from build123d import *

# Parameters (mm, degrees)
SKETCH1_W           = 30
SKETCH1_H           = 75
BOSS_EXTRUDE1_DEPTH = 12
CUT_EXTRUDE1_DEPTH  = 12
LPATTERN1_COUNT     = 3
LPATTERN1_PITCH     = 20
BOUNDARY2_START     = -15
BOUNDARY2_DEPTH     = 5


# Read off the part's stored shape, not the designer's step: Boundary2
with BuildPart() as part:
    # Sketch1 → Boss-Extrude1 (new body)
    with BuildSketch(Plane(origin=(0, 0, 0), x_dir=(1, 0, 0), z_dir=(0, 1, 0))):
        with Locations((15, 37.5)):
            Rectangle(SKETCH1_W, SKETCH1_H)
    extrude(amount=BOSS_EXTRUDE1_DEPTH)

    # Sketch3 → Cut-Extrude1 (cut)
    with BuildSketch(Plane(origin=(0, 0, 0), x_dir=(1, 0, 0), z_dir=(0, 1, 0))):
        Polygon((0, 5), (22.5, 12.5), (0, 20), align=None)
    cut_extrude1 = extrude(amount=CUT_EXTRUDE1_DEPTH, mode=Mode.SUBTRACT)

    # LPattern1: Cut-Extrude1 ×3
    with Locations(*[(0, 0, -i * LPATTERN1_PITCH) for i in range(1, LPATTERN1_COUNT)]):
        add(cut_extrude1, mode=Mode.SUBTRACT)

    # Boundary2 outline → Boundary2 (add)
    with BuildSketch(Plane.XY.offset(BOUNDARY2_START)):
        Polygon((30, 0), (25, 0), (30, -2), align=None)
    extrude(amount=BOUNDARY2_DEPTH)


solid = part.part
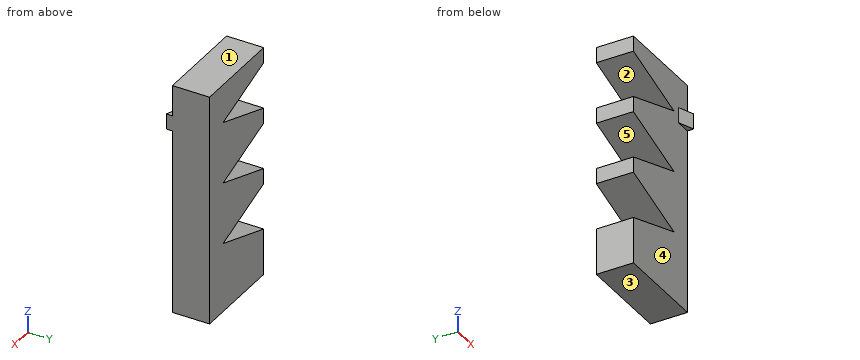
Input: part model. Units: mm. Frame: model coordinates. Face numbers are marked on the shaded views. A direction names the side the tool comes from. Coordinates: 2 decimals unless noted, no trailing zeros. Loops run counter-clockwise (first coordinate to the right, second up) from the corner with the lowest first, then second, coordinate; pieces in that order, holes last. Notation, with made-up numbers: (-5.75, 39) - (15.25, 39) arc R18 ccw to (15.25, 61) - close; hole circle Ø2 at (-8, -10.75). An arc over 180 degrees is marked (long way). Answer in a Markdown table with one row per item. Add a question column.
Item 1: Section query D-D on z = -11. Return the cut outline in (x, y), then the cut area to 3 significant figures.
Item 2: Mould query, pull axis Z, two halves, no side actions, for the marked faces 3, 4 and 5. Classes: released by +Z, released by -Z, zero draft, split by the parting line, or undercut.
Item 3: Contact query for flat-ended pins moving along their axis: P1, Ø4, axis at x = 26, y = 3.5, coming from the +Z side; P2, Ø1, axis at x = 27, y = -1, coming from the +Z side; P3, Ø4, axis at x = 4, z = -22, coming from the -Y side; P4, Ø1, axis at x = 26.5, y = -1, coming from the -Z side. Output: stop coordinate, or through.
Item 4: Section query B-B on x = 27.5. Return the cut outline in (y, z).
Item 5: Access query for the marked faces 1 and 2. Directions: +Z, -Z, +X, -X, +Y, -Y. A direction counts if a zero-diameter tool reaches every point of the face in a straight line with its end or side. Return the directions, or none.
Item 6: Section query C-C on y = 9.25. Return the cut outline in (x, z).
Item 7: Section query A-A on x = 13.5. Return the cut outline in (y, z).
Item 8: Line query: line 1 along Z through (x, y) = (22, 9.75); line 2 along Z through (x, y) = (12.5, 7); line 3 along Y through (x, z) = (19.75, -18.5). Output: solid intervals per line, ascending. Write a range as [from, to].
Recorded:
| question | item | result |
|---|---|---|
| 1 | outline | (18, 0) - (25, 0) - (30, -2) - (30, 12) - (18, 12) - close |
| 1 | area | 149 mm^2 |
| 2 | face 3 | released by -Z |
| 2 | face 4 | zero draft |
| 2 | face 5 | undercut |
| 3 | P1 | z = 0 |
| 3 | P2 | z = -10 |
| 3 | P3 | y = 0 |
| 3 | P4 | z = -15 |
| 4 | outline | (-1, -15) - (0, -15) - (0, -75) - (12, -75) - (12, 0) - (0, 0) - (0, -10) - (-1, -10) - close |
| 5 | face 1 | +Z, +X, -X, +Y, -Y |
| 5 | face 2 | -X, +Y, -Y |
| 6 | outline | (0, -75) - (30, -75) - (30, 0) - (0, 0) - (0, -5) - (22.5, -12.5) - (0, -20) - (0, -25) - (22.5, -32.5) - (0, -40) - (0, -45) - (22.5, -52.5) - (0, -60) - close |
| 7 | outline | (0, -75) - (12, -75) - (12, -55.5) - (0, -55.5) - close; (0, -49.5) - (12, -49.5) - (12, -35.5) - (0, -35.5) - close; (0, -29.5) - (12, -29.5) - (12, -15.5) - (0, -15.5) - close; (0, -9.5) - (12, -9.5) - (12, 0) - (0, 0) - close |
| 8 | line 1 | [-75, -52.67], [-52.33, -32.67], [-32.33, -12.67], [-12.33, 0] |
| 8 | line 2 | [-75, -55.83], [-49.17, -35.83], [-29.17, -15.83], [-9.17, 0] |
| 8 | line 3 | [0, 12] |
